Input: part model. Units: mm. Frame: model coordinates. A direction names the side the tool comes from. Coordinates: 2 decimals unless noted, no trailing zeros. Order: outer loops, then holes, each group sorted by start corner. A loop starts at its lowest first (then second) coordinate and runs counter-clockwise, first axis right, second up. Notation, with made-up numbers: (84.25, -2.5) -> (137.25, -2.5) arc R7 cw to (137.25, 3.5) -> close; hole circle Ø8 at (-14.75, 11.5). An arc over 180 degrees is marked (long way). Use one line per item in the form item = value. Start each with the question number.
1) Ray query, line 1 along X through (y, z) = (13, -3); line 2 along Y through (x, z) = (13.4, -11.5); line 3 along Z through (x, y) = (12.6, 2). Return the intervals inside material, ascending.
2) Section query C-C on z = 0. Output: boundary loops of the cut face in (x, y).
3) Section query B-B on y = 12.5. Output: boundary loops of the cut face in (x, z), then the cut area to 3 significant figures.
4) Section query D-D on z = -5. Output: boundary loops of the cut face in (x, y), then the cut area to 3 significant figures.
5) Section query A-A on z = -9. Output: boundary loops of the cut face in (x, y), then the cut area to 3 significant figures.
6) Access query for faces 4 (the cylindrical face through (13.373, -5.912, 8.394)), 5 (the flat face through (14.387, 0.2, -7.3)). Directions: +Z, -Z, +X, -X, +Y, -Y. A direction counts if a zero-diameter tool reaches every point of the face in a straight line with its end or side. Return the directions, or none.
7) Draft query along Y for faces 1 (the flat face through (12.387, 7, 0)), 2 (the cylindrical face through (13, 14, 0)), 3 (the cylindrical face through (13.373, 9.139, 14.334)). Return one class per face: pulls with the +Y half, pulls with the -Y half, needs draft (parallel to the pull), parting line crosses it, or undercut.
8) Pin query (flat end, axial travel): pin 1 (5 mm diameter, centred on y = -6, z = 10.39, fed in from -X); pin 2 (2 mm diameter, centred on x = 13.5, z = -4.5, fed in from +Y); pin 3 (4 mm diameter, centred on y = 7.5, z = -13, fed in from +X); pin 4 (1.5 mm diameter, centred on x = 14.5, y = 5.5, fed in from +Z). Return the tip coordinate at first contact, or that it passes through.
from build123d import *

# Parameters (mm, degrees)
SKETCH_2_R          = 2
CUT_EXTRUDE_1_DEPTH = 10
SKETCH_8_R          = 1.5
CUT_EXTRUDE_4_DEPTH = 10
SKETCH_9_R          = 1.5
CUT_EXTRUDE_5_DEPTH = 10


with BuildPart() as part:
    # 草图1 → 旋转1 (revolve)
    with BuildSketch(Plane.XY):
        with BuildLine():
            Line((14.38749457, 7), (14.38749457, 17))
            Line((14.38749457, 17), (12.38749457, 17))
            Line((12.38749457, 17), (12.38749457, 6.523034438))
            ThreePointArc((12.38749457, 6.523034438), (13.590896291, 3.359693142), (14, 0))
            Line((14, 0), (16, 0))
            ThreePointArc((16, 0), (15.591663047, 3.591663047), (14.38749457, 7))
        make_face()
    revolve(axis=Axis((0, 0, 0), (1, 0, 0)))

    # 草图2 → 切除-拉伸1 (cut)
    with BuildSketch(Plane.ZY.offset(-12.38749457)):
        with Locations((0, 12)):
            Circle(SKETCH_2_R)
        with Locations((10.392304845, -6)):
            Circle(SKETCH_2_R)
        with Locations((-10.392304845, -6)):
            Circle(SKETCH_2_R)
    extrude(amount=-CUT_EXTRUDE_1_DEPTH, mode=Mode.SUBTRACT)

    # 草图8 → 切除-拉伸4 (cut)
    with BuildSketch(Plane(origin=(18.259852425, 3.533095909, 0), x_dir=(0, 0, -1), z_dir=(0.9537169507482267, 0.30070579950427395, 0))):
        with Locations(Location((0, 0, 0), (0, 0, 90.000000005))):
            Circle(SKETCH_8_R)
    extrude(amount=-CUT_EXTRUDE_4_DEPTH, mode=Mode.SUBTRACT)

    # 草图9 → 切除-拉伸5 (cut)
    with BuildSketch(Plane(origin=(21.271029309, -4.482516334, 0), x_dir=(0, 0, -1), z_dir=(0.9537169507482268, -0.3007057995042737, 0))):
        with Locations(Location((0, -2.121270065, 0), (0, 0, 270))):
            Circle(SKETCH_9_R)
    extrude(amount=-CUT_EXTRUDE_5_DEPTH, mode=Mode.SUBTRACT)


solid = part.part
Answers below:
q1.line_1 = 12.39 to 14.39
q1.line_2 = -12.52 to -7.67, -4.33 to 12.52
q1.line_3 = -16.88 to -5.77, 5.77 to 16.88
q2.outline = (12.39, -17) -> (14.39, -17) -> (14.39, -7) arc R16 ccw to (14.74, -6.22) -> (12.82, -5.62) arc R14 cw to (12.39, -6.52) -> close; (12.39, 6.52) arc R14 cw to (13.53, 3.61) -> (15.43, 4.22) arc R16 ccw to (14.39, 7) -> (14.39, 10) -> (12.39, 10) -> close; (12.39, 14) -> (14.39, 14) -> (14.39, 17) -> (12.39, 17) -> close; (13.73, -2.76) -> (15.64, -3.36) arc R16 ccw to (15.95, 1.23) -> (13.99, 0.61) arc R14 cw to start
q3.outline = (12.39, -11.52) -> (14.39, -11.52) -> (14.39, -1.94) -> (12.39, -1.94) -> close; (12.39, 1.94) -> (14.39, 1.94) -> (14.39, 11.52) -> (12.39, 11.52) -> close
q3.area = 38.3 mm^2
q4.outline = (12.39, -16.25) -> (14.39, -16.25) -> (14.39, -4.9) arc R15.2 ccw to (14.39, 4.9) -> (14.39, 16.25) -> (12.39, 16.25) -> (12.39, 4.19) arc R13.08 cw to (12.39, -4.19) -> close
q4.area = 66.4 mm^2
q5.outline = (12.39, -14.42) -> (14.39, -14.42) -> (14.39, -7.44) -> (12.39, -7.44) -> close; (12.39, -4.56) -> (14.39, -4.56) -> (14.39, 14.42) -> (12.39, 14.42) -> close
q5.area = 51.9 mm^2
q6.face_4 = +X, -X
q6.face_5 = +X
q7.face_1 = needs draft
q7.face_2 = undercut
q7.face_3 = parting line crosses it
q8.pin_1 = 12.39
q8.pin_2 = 16.64
q8.pin_3 = 14.39
q8.pin_4 = 16.32
